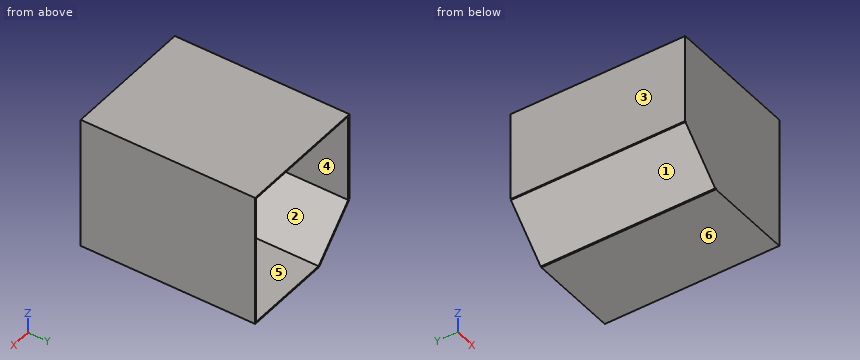
from build123d import *

# Parameters (mm, degrees)
BOSS_EXTRUDE1_DEPTH = 300
BOSS_EXTRUDE2_DEPTH = 2.5


with BuildPart() as part:
    # Sketch1 → Boss-Extrude1 (new body)
    with BuildSketch(Plane(origin=(0, 0, 0), x_dir=(1, 0, 0), z_dir=(0, 1, 0))):
        Polygon((-41.767766953, 114.267766953), (-114.267766953, 41.767766953), (-112.770991517, 40.270991517), (-112.877581569, 40), (-115, 40), (-115, -115), (115, -115), (115, 115), (-40, 115), (-40, 113.078362506), (-40.344526552, 112.844526552), align=None)
        Polygon((-112.5, -112.5), (112.5, -112.5), (112.5, 112.5), (-40, 112.5), (-112.5, 40), align=None, mode=Mode.SUBTRACT)
    extrude(amount=BOSS_EXTRUDE1_DEPTH)

    # Sketch2 → Boss-Extrude2 (add)
    with BuildSketch(Plane.XZ):
        Polygon((115, -115), (115, 115), (-115, 115), (-115, -40), (-112.877581569, -40), (-112.770991517, -40.270991517), (-114.267766953, -41.767766953), (-41.767766953, -114.267766953), (-40.344526552, -112.844526552), (-40, -113.078362506), (-40, -115), align=None)
    extrude(amount=BOSS_EXTRUDE2_DEPTH)


solid = part.part
Check sheet for the modelled part. Datum: model origin and axes. Units: mm. Face numbers are marked on the shaded views. A direction names the side the tool comes from. Round coordinates to 2 decimals unless told otherwise and drop trailing zeros. Loops run counter-clockwise (first coordinate to the right, second up) from the corner with the lowest first, then second, coordinate; pieces in that order, holes last. Notation, with made-up numbers: (64, 76) -> (123, 76) arc R7 ccw to (123, 81) -> close; hole circle Ø9 at (-35, 84). An arc over 180 degrees is marked (long way). Put each result on its own line as item: value. Start each with the question number.
1. Draft check along Z on the marked faces 3, 4, 5 and 6. Enter one of: +Z half, -Z half, draft (parallel to the pull), parting line (faces both ways), or undercut.
2. Access from +Z, -Z, +X, -X, +Y, -Y to the whole of each face (thin tool, end or side, straight path). Record for the marked faces 1 and 2.
3. Section check A-A (y = 276.5). Enter the section's corners in (x, z), plus the area to 3 significant figures.
4. Section check B-B (z = 16). Enter the section's corners in (x, y), plus the area to 4 significant figures.
5. Gauge pin test, flat ends, axial feed: pin 1 (2.5 mm diameter, centred on x = -114, y = 152.5, fed in from -Z); pin 2 (8 mm diameter, centred on x = -2.5, z = 29.5, fed in from +Y); pin 3 (1.5 mm diameter, centred on y = 130.5, z = -114.5, fed in from -X). Record the tip position at first contact, or that the pin passes through.
6. Scan lines: probe 1 along Z at (x, y) = (-6, 102); probe 2 along Y at (x, z) = (93.5, 106.5). Record each from-to range of solid material in increasing order.
7. Section check C-C (x = 25.5). Enter the section's corners in (y, z), plus the area to 4 significant figures.
Findings:
1. face 3: draft
1. face 4: undercut
1. face 5: undercut
1. face 6: -Z half
2. face 1: -Z, -X, +Y, -Y
2. face 2: +Y
3. outline: (-115, -40) -> (-112.88, -40) -> (-112.77, -40.27) -> (-114.27, -41.77) -> (-41.77, -114.27) -> (-40.34, -112.84) -> (-40, -113.08) -> (-40, -115) -> (115, -115) -> (115, 115) -> (-115, 115) -> close; hole (-112.5, -40) -> (-40, -112.5) -> (112.5, -112.5) -> (112.5, 112.5) -> (-112.5, 112.5) -> close
3. area: 2,160 mm^2
4. outline: (-115, -2.5) -> (115, -2.5) -> (115, 300) -> (112.5, 300) -> (112.5, 0) -> (-112.5, 0) -> (-112.5, 300) -> (-115, 300) -> close
4. area: 2,075 mm^2
5. pin 1: stops at z = -43.29
5. pin 2: stops at y = 0
5. pin 3: stops at x = -42.29
6. probe 1: z = -115 to -112.5, 112.5 to 115
6. probe 2: y = -2.5 to 0
7. outline: (-2.5, -115) -> (300, -115) -> (300, -112.5) -> (0, -112.5) -> (0, 112.5) -> (300, 112.5) -> (300, 115) -> (-2.5, 115) -> close
7. area: 2,075 mm^2
